```python
from build123d import *

# Parameters (mm, degrees)
ESQUISSE1_W             = 11.5
ESQUISSE1_H             = 9.8
BOSS_EXTRU_1_DEPTH      = 11
ESQUISSE2_W             = 9.5
ESQUISSE2_H             = 7.8
ENL_V_MAT_EXTRU_1_DEPTH = 10
ESQUISSE3_W             = 7.5
ESQUISSE3_H             = 3
ENL_V_MAT_EXTRU_2_DEPTH = 1
CONG_1_R                = 0.75
ESQUISSE4_W             = 11.5
ESQUISSE4_H             = 14.8
BOSS_EXTRU_2_DEPTH      = 1.5
ESQUISSE5_W             = 11.5
ESQUISSE5_H             = 1.25
BOSS_EXTRU_3_DEPTH      = 8
CONG_2_R                = 0.5


with BuildPart() as part:
    # Esquisse1 → Boss.-Extru.1 (new body)
    with BuildSketch(Plane.XY):
        with Locations((5.75, 4.9)):
            Rectangle(ESQUISSE1_W, ESQUISSE1_H)
    extrude(amount=BOSS_EXTRU_1_DEPTH)

    # Esquisse2 → Enlèv. mat.-Extru.1 (cut)
    with BuildSketch(Plane.XY.offset(11)):
        with Locations((5.75, 4.9)):
            Rectangle(ESQUISSE2_W, ESQUISSE2_H)
    extrude(amount=-ENL_V_MAT_EXTRU_1_DEPTH, mode=Mode.SUBTRACT)

    # Esquisse3 → Enlèv. mat.-Extru.2 (cut)
    with BuildSketch(Plane(origin=(0, 9.8, 0), x_dir=(1, 0, 0), z_dir=(0, 1, 0))):
        with Locations((5.75, -1.5)):
            Rectangle(ESQUISSE3_W, ESQUISSE3_H)
    extrude(amount=-ENL_V_MAT_EXTRU_2_DEPTH, mode=Mode.SUBTRACT)

    # Congé1
    cong_1_edges = [part.edges().sort_by_distance(p)[0] for p in [
        (5.75, 8.8, 1),
        (5.75, 8.8, 3),
    ]]
    fillet(cong_1_edges, radius=CONG_1_R)

    # Esquisse4 → Boss.-Extru.2 (add)
    with BuildSketch(Plane(origin=(0, 0, 0), x_dir=(-1, 0, 0), z_dir=(0, 0, -1))):
        with Locations((-5.75, 4.9)):
            Rectangle(ESQUISSE4_W, ESQUISSE4_H)
    extrude(amount=BOSS_EXTRU_2_DEPTH)

    # Esquisse5 → Boss.-Extru.3 (add)
    with BuildSketch(Plane(origin=(0, 0, -1.5), x_dir=(-1, 0, 0), z_dir=(0, 0, -1))):
        with Locations((-5.75, 11.675)):
            Rectangle(ESQUISSE5_W, ESQUISSE5_H)
        with Locations((-5.75, -1.875)):
            Rectangle(ESQUISSE5_W, ESQUISSE5_H)
    extrude(amount=BOSS_EXTRU_3_DEPTH)

    # Congé2
    cong_2_edges = [part.edges().sort_by_distance(p)[0] for p in [
        (5.75, -2.5, 0),
        (5.75, 12.3, 0),
    ]]
    fillet(cong_2_edges, radius=CONG_2_R)


solid = part.part
```
Geometry: final body of the model. Coordinates: model frame, mm. A direction names the side the tool comes from. Give positions to 0.01 mm unless a question says otherwise; leave off trailing zeros. Loops run counter-clockwise (first coordinate to the right, second up) from the corner with the lowest first, then second, coordinate; pieces in that order, holes last. Notation, with made-up numbers: (-32, -13.75) -> (7, -13.75) arc R24 cw to (7, 16.25) -> close; hole circle Ø4 at (-4.5, 47). An arc over 180 degrees is marked (long way). Return JSON: item names as keys, results as strings.
Item 1: Mould query, pull axis X, two halves, no side actions, for faces 4 (the flat face through (6, 1, 6)), 5 (the flat face through (0, 5, 3)), 6 (the flat face through (6, -2.5, -5)), 7 (the flat face through (9.5, 9, 1)). Classes: released by +X, released by -X, zero draft, split by the parting line, or undercut.
Filled in:
{"face 4": "undercut", "face 5": "released by -X", "face 6": "zero draft", "face 7": "undercut"}
Item 2: Section C-C, the plane x = 1.25. Output: boundary loops of the cut face in (y, z), plus the area to 3 significant figures.
Filled in:
{"outline": "(-2.5, -9.5) -> (-1.25, -9.5) -> (-1.25, -1.5) -> (11.05, -1.5) -> (11.05, -9.5) -> (12.3, -9.5) -> (12.3, -0.5) arc R0.5 ccw to (11.8, 0) -> (9.8, 0) -> (9.8, 11) -> (8.8, 11) -> (8.8, 1) -> (1, 1) -> (1, 11) -> (0, 11) -> (0, 0) -> (-2, 0) arc R0.5 ccw to (-2.5, -0.5) -> close", "area": "71.9 mm^2"}
Item 3: Pin query (flat end, axial travel): P1, Ø6, axis at x = 4.5, y = 2.5, coming from the -Z side; P2, Ø4, axis at y = 3, z = -5, coming from the -X side; P3, Ø3.5, axis at x = 3.5, z = 3, coming from the +Y side; P4, Ø3, axis at x = 3, y = 3.5, coming from the +Z side. Return the tip coordinate at first contact, or that it passes through.
Filled in:
{"P1": "z = -1.5", "P2": "through", "P3": "y = 9.8", "P4": "z = 1"}
Item 4: Section A-A, the plane z = -4.5. Output: boundary loops of the cut face in (x, y).
Filled in:
{"outline": "(0, -2.5) -> (11.5, -2.5) -> (11.5, -1.25) -> (0, -1.25) -> close; (0, 11.05) -> (11.5, 11.05) -> (11.5, 12.3) -> (0, 12.3) -> close"}
Item 5: Section B-B, the plane y = 8.5. Output: boundary loops of the cut face in (x, z).
Filled in:
{"outline": "(0, -1.5) -> (11.5, -1.5) -> (11.5, 11) -> (10.5, 11) -> (10.5, 1) -> (9.5, 1) -> (9.5, 0.85) -> (2, 0.85) -> (2, 1) -> (1, 1) -> (1, 11) -> (0, 11) -> close"}
Item 6: Section D-D, the plane x = 8.75. Output: boundary loops of the cut face in (y, z), plus the area to 3 significant figures.
Filled in:
{"outline": "(-2.5, -9.5) -> (-1.25, -9.5) -> (-1.25, -1.5) -> (11.05, -1.5) -> (11.05, -9.5) -> (12.3, -9.5) -> (12.3, -0.5) arc R0.5 ccw to (11.8, 0) -> (8.8, 0) -> (8.8, 0.25) arc R0.75 ccw to (8.05, 1) -> (1, 1) -> (1, 11) -> (0, 11) -> (0, 0) -> (-2, 0) arc R0.5 ccw to (-2.5, -0.5) -> close; (8.8, 3.75) arc R0.75 ccw to (9.55, 3) -> (9.8, 3) -> (9.8, 11) -> (8.8, 11) -> close", "area": "68.7 mm^2"}
Item 7: Line query: line 1 (X direction, y = 2.5, z = 8.5); line 2 (Y direction, x = 3, z = -3); line 3 (Y direction, x = 8.5, z = 7.25). Output: solid intervals per line, ascending.
Filled in:
{"line 1": "0 to 1, 10.5 to 11.5", "line 2": "-2.5 to -1.25, 11.05 to 12.3", "line 3": "0 to 1, 8.8 to 9.8"}
Item 8: Access query for faces 1 (the flat face through (6, 5, -1.5)), 2 (the flat face through (1, 5, 6)), 3 (the flat face through (6, 9.8, 7)). Directions: +Z, -Z, +X, -X, +Y, -Y. A direction counts if a zero-diameter tool reaches every point of the face in a straight line with its end or side. Return the directions, or none.
Filled in:
{"face 1": "-Z, +X, -X", "face 2": "+Z", "face 3": "+Z, +X, -X, +Y"}
